Autodesk Inventor part; units mm, degrees
ref_plane "YZ Plane" through (0, 0, 0) normal (1, 0, 0) x (0, 1, 0)
ref_plane "XZ Plane" through (0, 0, 0) normal (0, 1, 0) x (-1, 0, 0)
ref_plane "XY Plane" through (0, 0, 0) normal (0, 0, 1) x (1, 0, 0)
sketch "Sketch1" plane through (0, 0, 0) normal (1, 0, 0) x (0, 1, 0)
  line L0 (10.3439, 0) -> (-10.3439, 0) construction
  line L1 (8.828, -17.5) -> (-11.172, -17.5)
  line L2 (8.828, -17.5) -> (8.828, -23)
  line L3 (8.828, -23) -> (1.828, -23)
  line L4 (1.828, -23) -> (1.828, -34.8153)
  line L5 (1.828, -34.8153) -> (-4.172, -34.8153)
  line L6 (-4.172, -34.8153) -> (-4.172, -23)
  line L7 (-4.172, -23) -> (-11.172, -23)
  line L8 (-11.172, -23) -> (-11.172, -17.5)
  line L9 (0, 48.9131) -> (0, -72.8322) construction
  point P0 (0, 0)
  point P1 (0, 0)
  dimension "d0" = 35
  dimension "d1" = 5.5
  dimension "d2" = 6
  dimension "d3" = 7
revolve "Revolution1" add sketch "Sketch1" angle 360 about axis through (0, 10.3439, 0) along (0, -1, 0)
sketch "Sketch2" plane through (0, 0, 0) normal (1, 0, 0) x (0, 1, 0)
  line L0 (1.828, 34.8153) -> (1.828, -34.8153)
  line L1 (-4.172, 34.8153) -> (-4.172, -34.8153)
  line L2 (1.828, 34.8153) -> (1.828, -34.8153)
  line L3 (-4.172, 34.8153) -> (-4.172, -34.8153)
  line L4 (1.828, 34.8153) -> (1.828, -34.8153)
  line L5 (-4.172, 34.8153) -> (-4.172, -34.8153)
  line L6 (1.828, 34.8153) -> (1.828, -34.8153) construction
  line L7 (-4.172, 34.8153) -> (-4.172, -34.8153) construction
  line L8 (1.828, 34.8153) -> (1.828, -34.8153) construction
  line L9 (-4.172, 34.8153) -> (-4.172, -34.8153) construction
  line L10 (1.828, 34.8153) -> (1.828, -34.8153) construction
  line L11 (-4.172, 34.8153) -> (-4.172, -34.8153) construction
  line L12 (0.828, -33.5153) -> (1.828, -34.8153) construction
  line L13 (1.828, -34.8153) -> (-0.172, -34.8153) construction
  line L14 (-0.172, -34.8153) -> (0.828, -33.5153) construction
  line L15 (0.828, -34.8153) -> (0.828, -33.5153) construction
  line L16 (1.828, -34.8153) -> (-4.172, -34.8153) construction
  line L17 (0.828, -33.5153) -> (1.828, -34.8153)
  line L18 (-0.172, -34.8153) -> (1.828, -34.8153)
  line L19 (0.828, -33.5153) -> (-0.172, -34.8153)
  point P0 (0, 0)
  dimension "d5" = 1.3
  dimension "d6" = 2
sketch "Sketch3" plane through (0, 0, 0) normal (0, 0, 1) x (1, 0, 0)
  point P0 (0, 0)
sketch "Sketch4" plane through (0, 0, 0) normal (1, 0, 0) x (0, 1, 0)
  line L0 (14.7871, 0) -> (-17.2316, 0)
  point P0 (0, 0)
revolve "Revolution2" cut sketch "Sketch2" angle 360 about axis through (0, 14.7871, 0) along (0, -1, 0)
pattern_linear "Rectangular Pattern1" count 4 spacing 2 along (0, -1, 0) of "Revolution2"
properties part number "34_Vong_chan_dau"
Geometry check sheet. Reference: the model listing, model coordinates, mm. A direction names the side the tool comes from. Give positions to 0.01 mm unless a question says otherwise; leave off trailing zeros. Write each loop counter-clockwise with the first axis right and the second up, starting at its lowest first coordinate (ties: lowest second). Pieces come first, ordered by that corner, then holes.
1) Material ranges on L1, parallel to X at y = -6.5, z = 0; L2, parallel to X at y = -3.25, z = -24.5; L3, parallel to Y at x = 10.5, z = 24, recorded low to high.
2) Gauge pin test, flat ends, axial feed: pin 1 (4 mm diameter, centred on x = -8.5, y = -3.5, fed in from -Z); pin 2 (1.5 mm diameter, centred on x = -1, z = 25, fed in from +Y); pin 3 (1.5 mm diameter, centred on x = 16.5, y = 3, fed in from +Z); pin 4 (21 mm diameter, centred on x = 0, z = 0, fed in from +Y). Record the tip position at first contact, or that the pin passes through.
3) Section check B-B, the plane x = 0. Record the boundary of the cut face in (y, z).
4) Section check C-C, the plane y = -8.75. Record the boundary of the cut face in (x, z), and give its area (3 significant figures).
5) Access from +Z, -Z, +X, -X, +Y, -Y to the whole of each face (thin tool, end or side, straight path). Record for faces 1 (the cylindrical face through (-10.648, -1.312, 13.887)), 2 (the cylindrical face through (22.804, 5.279, 2.994)), 3 (the flat face through (-7, -4.172, -23)).
6) Section check A-A, the plane z = 0. Record the boundary of the cut face in (x, y), and give its area (3 significant figures).
Computed:
1. L1: x = -23 to -17.5, 17.5 to 23
1. L2: x = -23.02 to 23.02
1. L3: y = -4.17 to 1.83
2. pin 1: stops at z = -34.18
2. pin 2: stops at y = 1.83
2. pin 3: stops at z = 16.76
2. pin 4: passes through
3. outline: (-11.17, -23) - (-4.17, -23) - (-4.17, -34.82) - (-3.17, -33.52) - (-2.17, -34.82) - (-1.17, -33.52) - (-0.17, -34.82) - (0.83, -33.52) - (1.83, -34.82) - (1.83, -23) - (8.83, -23) - (8.83, -17.5) - (-11.17, -17.5) - close; (-11.17, 17.5) - (8.83, 17.5) - (8.83, 23) - (1.83, 23) - (1.83, 34.82) - (0.83, 33.52) - (-0.17, 34.82) - (-1.17, 33.52) - (-2.17, 34.82) - (-3.17, 33.52) - (-4.17, 34.82) - (-4.17, 23) - (-11.17, 23) - close
4. outline: circle Ø46 at (0, 0); hole circle Ø35 at (0, 0)
4. area: 700 mm2
5. face 1: +Y, -Y
5. face 2: +Y
5. face 3: -Y
6. outline: (-34.82, -4.17) - (-23, -4.17) - (-23, -11.17) - (-17.5, -11.17) - (-17.5, 8.83) - (-23, 8.83) - (-23, 1.83) - (-34.82, 1.83) - (-33.52, 0.83) - (-34.82, -0.17) - (-33.52, -1.17) - (-34.82, -2.17) - (-33.52, -3.17) - close; (17.5, -11.17) - (23, -11.17) - (23, -4.17) - (34.82, -4.17) - (33.52, -3.17) - (34.82, -2.17) - (33.52, -1.17) - (34.82, -0.17) - (33.52, 0.83) - (34.82, 1.83) - (23, 1.83) - (23, 8.83) - (17.5, 8.83) - close
6. area: 354 mm2
